Can you work these out from the model? Positions are in its coordinate system, mm. A direction names the side the tool comes from. Coordinates: 2 decimals unless noted, no trailing zeros. Order: outer loops, then holes, each group sorted by start corner. A loop starts at its lowest first (then second) coordinate and runs counter-clockwise, first axis right, second up. Notation, with made-up numbers: (-28.75, 73) -> (12.25, 73) arc R24 cw to (12.25, 102) -> close; hole circle Ø2 at (77, 24.5). An arc over 180 degrees is marked (long way). Answer as a JSON object with one key per item and string values. Group by question number.
(1) For pin 1 (5 mm diameter, centred on x = 25, z = -14.5, fed in from +Y); pin 2 (0.7 mm diameter, centred on y = 2.5, z = -10.5, fed in from +X), each with a flat end and sliding along its axis, tell me the tip position at first contact or that it passes through.
(2) I want a section at C-C, the plane y = 0.9. State how many separate pieces and enclosed holes the cut face has, plus the area to 3 significant figures.
(3) I want a section at B-B, the plane y = 3.05. List the corners of the cut face in (x, z) for me (3 decimals).
(4) I want a section at A-A, the plane z = -20.5. List the corners of the cut face in (x, y) for me, plus the area to 3 significant figures.
(5) If we mould it in two halves opening along Z, with no side actions, what happens to faces 4 (the cylindrical face through (0.526, 2.028, -38.001)), 5 (the flat face through (14, 2, 0)), 6 (the flat face through (24, 3, -17.393)), 7 (the flat face through (26.75, 2, -4))? For each: pulls with the +Z half, pulls with the -Z half, needs draft (parallel to the pull), parting line crosses it, or undercut.
(6) Which directions (+Z, -Z, +X, -X, +Y, -Y) give clear straight access to the entire face, cutting with the end or side of a thin tool? Please do faces 1 (the flat face through (9.026, 2.986, -31.007)), 2 (the cylindrical face through (8.99, 0.986, -30.086)), 3 (the flat face through (20.75, 3, -12)).
(7) I need wall thicknesses on line 1 (Z direction, x = 21.5, y = 2.1); line 2 (X direction, y = 2, z = -11.5). Which ranges of each line are inside material? Lowest first, please.
from build123d import *

# Parameters (mm, degrees)
BOSS_EXTRUDE1_DEPTH = 4
SKETCH2_W           = 9.844621866
SKETCH2_H           = 0.8
CUT_EXTRUDE1_DEPTH  = 6
SKETCH3_W           = 9.843082996
SKETCH3_H           = 1.6
CUT_EXTRUDE2_DEPTH  = 6
SKETCH5_R           = 1.6
CUT_EXTRUDE4_DEPTH  = 4
FILLET1_R           = 1.75
SKETCH10_R          = 1.85
CUT_EXTRUDE7_DEPTH  = 4
CAVITY2_START       = 2
CAVITY2_OUTLINE_R   = 1.85
CAVITY2_DEPTH       = 3


with BuildPart() as part:
    # Sketch1 → Boss-Extrude1 (new body)
    with BuildSketch(Plane(origin=(0, 0, 0), x_dir=(1, 0, 0), z_dir=(0, 1, 0))):
        Polygon((26.75, 16.194621866), (26.75, 38.5), (0, 38.5), (0, 0), (26.75, 0), (26.75, 8.75), (21.35, 8.75), (21.35, 16.194621866), align=None)
    extrude(amount=BOSS_EXTRUDE1_DEPTH)

    # Sketch2 → Cut-Extrude1 (cut)
    with BuildSketch(Plane(origin=(26.75, 0, 0), x_dir=(0, 0, -1), z_dir=(1, 0, 0))):
        with Locations((12.472310933, 2)):
            Rectangle(SKETCH2_W, SKETCH2_H)
    extrude(amount=-CUT_EXTRUDE1_DEPTH, mode=Mode.SUBTRACT)

    # Sketch3 → Cut-Extrude2 (cut)
    with BuildSketch(Plane(origin=(26.75, 0, 0), x_dir=(0, 0, -1), z_dir=(1, 0, 0))):
        with Locations((12.471541498, 3.2)):
            Rectangle(SKETCH3_W, SKETCH3_H)
    extrude(amount=-CUT_EXTRUDE2_DEPTH, mode=Mode.SUBTRACT)

    # Sketch5 → Cut-Extrude4 (cut)
    with BuildSketch(Plane(origin=(0, 4, 0), x_dir=(1, 0, 0), z_dir=(0, 1, 0))):
        with Locations(Location((7.307, 20.085, 0), (0, 0, 270))):
            Circle(SKETCH5_R)
    extrude(amount=-CUT_EXTRUDE4_DEPTH, mode=Mode.SUBTRACT)

    # Chamfer1: read off the stored shape, not the designer's step
    # Chamfer1: loft between two sections, ruled curve by curve
    chamfer1_from = [
        Edge.make_line((21.35, 1.5, -16.194621866), (21.35, 1.5, -8.75)),
        Edge.make_line((21.35, 1.5, -8.75), (26.75, 1.5, -8.75)),
        Edge.make_line((21.35, 1.5, -16.194621866), (26.75, 1.5, -16.194621866)),
        Edge.make_line((26.75, 1.5, -16.194621866), (26.75, 1.5, -8.75)),
    ]
    chamfer1_to = [
        Edge.make_line((19.85, 0, -17.694621866), (19.85, 0, -7.25)),
        Edge.make_line((19.85, 0, -7.25), (26.75, 0, -7.25)),
        Edge.make_line((19.85, 0, -17.694621866), (26.75, 0, -17.694621866)),
        Edge.make_line((26.75, 0, -17.694621866), (26.75, 0, -7.25)),
    ]
    chamfer1 = Solid(Shell([*[Face.make_surface_from_curves(chamfer1_from[k], chamfer1_to[k]) for k in range(4)], Face(Wire(chamfer1_from)), Face(Wire(chamfer1_to))]))
    add(chamfer1, mode=Mode.SUBTRACT)

    # Fillet1
    fillet1_edges = [part.edges().sort_by_distance(p)[0] for p in [
        (0, 2, -38.5),
        (0, 2, 0),
    ]]
    fillet(fillet1_edges, radius=FILLET1_R)

    # Sketch10 → Cut-Extrude7 (cut)
    with BuildSketch(Plane(origin=(0, 0, 0), x_dir=(-1, 0, 0), z_dir=(0, -1, 0))):
        with Locations(Location((-8.434644349, 28.321384576, 0), (0, 0, 90))):
            Circle(SKETCH10_R)
    extrude(amount=-CUT_EXTRUDE7_DEPTH, mode=Mode.SUBTRACT)

    # Cavity2: read off the stored shape, not the designer's step
    # Cavity2 outline → Cavity2 (cut)
    with BuildSketch(Plane(origin=(0, 0, 0), x_dir=(1, 0, 0), z_dir=(0, 1, 0)).offset(CAVITY2_START)):
        Polygon((11.54125505, 27.663886828), (10.557359451, 30.683039489), (7.450748751, 31.340537236), (5.328033648, 28.978882323), (6.311929246, 25.959729663), (9.418539947, 25.302231916), align=None)
        with Locations((8.434644349, 28.321384576)):
            Circle(CAVITY2_OUTLINE_R, mode=Mode.SUBTRACT)
    extrude(amount=CAVITY2_DEPTH, mode=Mode.SUBTRACT)


solid = part.part
Computed values:
{
 "1": {"pin 1": "stops at y = 1.6", "pin 2": "stops at x = 20.75"},
 "2": {"separate pieces": "1", "enclosed holes": "2", "area": "958 mm2"},
 "3": {"outline": "(0, -36.75) arc R1.75 ccw to (1.75, -38.5) -> (26.75, -38.5) -> (26.75, -17.393) -> (20.75, -17.393) -> (20.75, -7.55) -> (26.75, -7.55) -> (26.75, 0) -> (1.75, 0) arc R1.75 ccw to (0, -1.75) -> close; hole (5.328, -28.979) -> (7.451, -31.341) -> (10.557, -30.683) -> (11.541, -27.664) -> (9.419, -25.302) -> (6.312, -25.96) -> close; hole circle Ø3.2 at (7.307, -20.085)"},
 "4": {"outline": "(0, 0) -> (5.76, 0) -> (5.76, 4) -> (0, 4) -> close; (8.85, 0) -> (26.75, 0) -> (26.75, 4) -> (8.85, 4) -> close", "area": "94.6 mm2"},
 "5": {"face 4": "pulls with the -Z half", "face 5": "pulls with the +Z half", "face 6": "undercut", "face 7": "needs draft"},
 "6": {"face 1": "+Y", "face 2": "+Y, -Y", "face 3": "+X, +Y"},
 "7": {"line 1": "z = -38.5 to -17.39, -7.55 to 0", "line 2": "x = 0 to 20.75"}
}
